Could you check a few things on this model? Use its own coordinates, in mm. A direction names the side the tool comes from. Give positions to 0.01 mm unless a question says otherwise; leave off trailing zeros. Loops run counter-clockwise (first coordinate to the right, second up) from the corner with the lowest first, then second, coordinate; pieces in that order, holes last. Notation, with made-up numbers: (50, 55.5) -> (91, 55.5) arc R9 cw to (91, 68.5) -> close; hole circle Ø9 at (-29.75, 83). An arc over 180 degrees is marked (long way). Put each result on its own line as item: value.
```python
from build123d import *

# Parameters (mm, degrees)
SKETCH_1_W          = 150
SKETCH_1_H          = 150
EXTRUDE_1_DEPTH     = 20
SKETCH_2_W          = 138
SKETCH_2_H          = 138
EXTRUDE_2_DEPTH     = 10
SKETCH_3_W          = 138
SKETCH_3_H          = 138
EXTRUDE_3_DEPTH     = 10
SKETCH_4_W          = 130
SKETCH_4_H          = 130
CUT_EXTRUDE_1_DEPTH = 114.357840488


with BuildPart() as part:
    # Эскиз1 → Бобышка-Вытянуть1 (new body)
    with BuildSketch(Plane(origin=(0, 0, 0), x_dir=(1, 0, 0), z_dir=(0, 1, 0))):
        Rectangle(SKETCH_1_W, SKETCH_1_H)
    extrude(amount=EXTRUDE_1_DEPTH)

    # Эскиз2 → Бобышка-Вытянуть2 (add)
    with BuildSketch(Plane(origin=(0, 20, 0), x_dir=(1, 0, 0), z_dir=(0, 1, 0))):
        Rectangle(SKETCH_2_W, SKETCH_2_H)
    extrude(amount=EXTRUDE_2_DEPTH)

    # Эскиз3 → Бобышка-Вытянуть3 (add)
    with BuildSketch(Plane(origin=(0, 0, 0), x_dir=(-1, 0, 0), z_dir=(0, -1, 0))):
        Rectangle(SKETCH_3_W, SKETCH_3_H)
    extrude(amount=EXTRUDE_3_DEPTH)

    # Эскиз4 → Вырез-Вытянуть1 (cut, through all)
    with BuildSketch(Plane(origin=(0, 30, 0), x_dir=(1, 0, 0), z_dir=(0, 1, 0))):
        Rectangle(SKETCH_4_W, SKETCH_4_H)
    extrude(amount=-CUT_EXTRUDE_1_DEPTH, mode=Mode.SUBTRACT)


solid = part.part
```
1. If we section it at B-B (y = -3): List the corners of the cut face in (x, z) for me, then the cut area to 3 significant figures.
Recorded:
outline: (-69, -69) -> (69, -69) -> (69, 69) -> (-69, 69) -> close; hole (-65, -65) -> (65, -65) -> (65, 65) -> (-65, 65) -> close
area: 2,140 mm^2
2. I need wall thicknesses on line 1 (X direction, y = 28, z = 23); line 2 (X direction, y = 11.5, z = 45.5). Which ranges of each line are inside material? Lowest first, please.
Recorded:
line 1: x = -69 to -65, 65 to 69
line 2: x = -75 to -65, 65 to 75
3. If we section it at A-A (x = -62): List the corners of the cut face in (y, z) for me.
Recorded:
outline: (-10, -69) -> (0, -69) -> (0, -75) -> (20, -75) -> (20, -69) -> (30, -69) -> (30, -65) -> (-10, -65) -> close; (-10, 65) -> (30, 65) -> (30, 69) -> (20, 69) -> (20, 75) -> (0, 75) -> (0, 69) -> (-10, 69) -> close
4. For faces 1 (the face through (1, -5, 69)), 2 (the face through (1, -5, -69)), 3 (the face through (65, 10, 1)), which set-ups out of +Z, -Z, +X, -X, +Y, -Y let a thin tool reach every point of the face, with its end or its side?
Recorded:
face 1: +Z, +X, -X, -Y
face 2: -Z, +X, -X, -Y
face 3: +Y, -Y
5. If we section it at C-C (z = 40): List the corners of the cut face in (x, y) for me, then the cut area to 3 significant figures.
Recorded:
outline: (-75, 0) -> (-69, 0) -> (-69, -10) -> (-65, -10) -> (-65, 30) -> (-69, 30) -> (-69, 20) -> (-75, 20) -> close; (65, -10) -> (69, -10) -> (69, 0) -> (75, 0) -> (75, 20) -> (69, 20) -> (69, 30) -> (65, 30) -> close
area: 560 mm^2
6. I'm going to push flat-ended pins straight in: pin 1 (1.5 mm diameter, centred on y = -4, z = 14.5, fed in from +X); pin 2 (5 mm diameter, centred on y = -1, z = 58, fed in from -X); pin 3 (3 mm diameter, centred on x = 27.5, y = 25.5, fed in from +Z); pin 4 (3 mm diameter, centred on x = 16, y = 25.5, fed in from -Z). Where does each tip first touch, or does it pass through?
Recorded:
pin 1: stops at x = 69
pin 2: stops at x = -75
pin 3: stops at z = 69
pin 4: stops at z = -69
7. Thinking about a two-plate mould opening in Z: for faces 4 (the face through (-65, 10, 1)), 5 (the face through (-1, 25, 69)), 6 (the face through (-75, 10, 1)), which applies, pulls with the +Z half, pulls with the -Z half, needs draft (parallel to the pull), parting line crosses it, or undercut?
Recorded:
face 4: undercut
face 5: pulls with the +Z half
face 6: needs draft
8. If we section it at D-D (y = 6): List the corners of the cut face in (x, z) for me, then the cut area to 3 significant figures.
Recorded:
outline: (-75, -75) -> (75, -75) -> (75, 75) -> (-75, 75) -> close; hole (-65, -65) -> (65, -65) -> (65, 65) -> (-65, 65) -> close
area: 5,600 mm^2
